Design review of the part built by this model. Coordinates are the model's own, in mm. Round coordinates to 2 decimals unless told otherwise and drop trailing zeros. Order: outer loops, then holes, each group sorted by start corner. A loop starts at its lowest first (then second) coordinate and runs counter-clockwise, first axis right, second up.
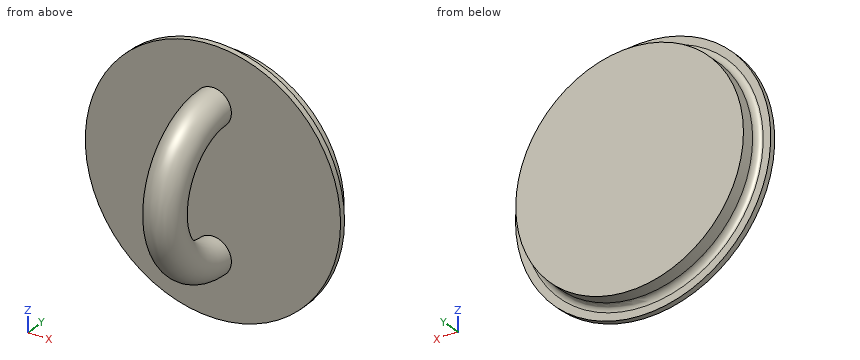
from build123d import *

# Parameters (mm, degrees)
SKETCH001_R         = 1.596485
REVOLUTION001_ANGLE = -180


with BuildPart() as part:
    # Sketch → Revolution (revolve)
    with BuildSketch(Plane.XY):
        with BuildLine():
            Line((0, 1.922073), (11.1, 1.922073))
            Line((11.1, 1.922073), (11.1, 2.422073))
            Line((11.1, 2.422073), (10.441024, 2.422073))
            ThreePointArc((9.9, 2.963097), (10.058462, 2.580535), (10.441024, 2.422073))
            Line((9.9, 2.963097), (9.9, 4.122073))
            Line((9.9, 4.122073), (0, 4.122073))
            Line((0, 4.122073), (0, 1.922073))
        make_face()
    revolve(axis=Axis((0, 0, 0), (0, 1, 0)))

    # Sketch001 (on Face3 of Revolution) → Revolution001 (revolve)
    with BuildSketch(Plane.XZ.offset(-1.922073)):
        with Locations((0.008299, -6.053004)):
            Circle(SKETCH001_R)
    revolve(axis=Axis((0, 1.922073, 0), (1, 0, 0)), revolution_arc=REVOLUTION001_ANGLE)


solid = part.part
1) Take a section at A-A on z = 0. Give the boundary of the cut face in (x, y), plus the area to 3 significant figures.
Results:
outline: (-11.1, 1.92) - (11.1, 1.92) - (11.1, 2.42) - (10.44, 2.42) arc R0.54 cw to (9.9, 2.96) - (9.9, 4.12) - (-9.9, 4.12) - (-9.9, 2.96) arc R0.54 cw to (-10.44, 2.42) - (-11.1, 2.42) - close; circle Ø3.19 at (0.01, -4.13)
area: 52.9 mm2
2) Clearance check with flat-ended pins moving along their axes: P1, Ø6.5, axis at x = -2, z = 0.5, coming from the -Y side; P2, Ø4, axis at x = 6.5, z = 5.5, coming from the -Y side; P3, Ø5, axis at y = -3.5, z = -4.5, coming from the -X side; P4, Ø5, axis at x = 3.5, y = -4, coming from the +Z side. State where each tip first meets the part, or that it passes through.
Results:
P1: stops at y = -5.73
P2: stops at y = 1.92
P3: stops at x = -1.59
P4: stops at z = 5.15
3) Take a section at B-B on x = 0. Give the boundary of the cut face in (y, z), plus the area to 3 significant figures.
Results:
outline: (1.92, -11.1) - (2.42, -11.1) - (2.42, -10.44) arc R0.54 cw to (2.96, -9.9) - (4.12, -9.9) - (4.12, 9.9) - (2.96, 9.9) arc R0.54 cw to (2.42, 10.44) - (2.42, 11.1) - (1.92, 11.1) - (1.92, 7.65) arc R7.65 ccw to (1.92, -7.65) - close; hole (1.92, -4.46) - (1.92, 4.46) arc R4.46 ccw to start
area: 106 mm2
4) To check wall thickness, follow line 1 along Y through (x, z) = (-6.5, 8.25); line 2 along Y through (x, z) = (-8.25, 0.5); line 3 along Z through (x, y) = (-0.5, 1.75). State the ranges of each line that lie inside material, in increasing order.
Results:
line 1: y = 1.92 to 2.42
line 2: y = 1.92 to 4.12
line 3: z = -7.56 to -4.54, 4.54 to 7.56
